Can you work these out from the model? Positions are in its coordinate system, mm. A direction names the side the tool comes from. Give positions to 0.01 mm unless a question says otherwise; leave off trailing zeros. Order: outer loops, then holes, each group sorted by start corner. A loop starts at its lowest first (then second) coordinate and runs counter-clockwise, first axis right, second up. Notation, with made-up numbers: (51, 73) - (104, 73) arc R33 ccw to (104, 110) - close; hole circle Ø10 at (29, 41.5). An arc over 180 degrees is marked (long way). Answer as CSV lines item,"result".
```python
from build123d import *

# Parameters (mm, degrees)
F0_W     = 62.4
F0_H     = 62.4
F0_W_2   = 60
F0_H_2   = 60
F1_DEPTH = 50


with BuildPart() as f1:
    # F0 (on Top) → F1 (new body)
    with BuildSketch(Plane.XY):
        Rectangle(F0_W, F0_H)
        Rectangle(F0_W_2, F0_H_2, mode=Mode.SUBTRACT)
    extrude(amount=F1_DEPTH)


solid = f1.part
```
1) I want a section at A-A on z = 23.5. Write out the boundary of the cut face in (x, y).
Answer block:
outline,"(-31.2, -31.2) - (31.2, -31.2) - (31.2, 31.2) - (-31.2, 31.2) - close; hole (-30, -30) - (30, -30) - (30, 30) - (-30, 30) - close"
2) If we mould it in two halves opening along Y, with no side actions, what happens to faces 3 (the flat face through (0, 30, 25)), 4 (the flat face through (-31.2, 0, 25)), 5 (the flat face through (-30, 0, 25)), 6 (the flat face through (0, -31.2, 25))? For each: +Y half, -Y half, draft (parallel to the pull), parting line (faces both ways), or undercut.
Answer block:
face 3,"undercut"
face 4,"draft"
face 5,"undercut"
face 6,"-Y half"
3) I'm going to push a flat-ended pin straight in: P1, Ø8, axis at x = -6.5, y = -22.5, coming from the +Z side. Where does the tip first touch, or does it pass through?
Answer block:
P1,"through"
4) I need wall thicknesses on line 1 along Y through (x, z) = (9, 10.5). Which ranges of the line are inside material? Lowest first, please. Write a range as [from, to].
Answer block:
line 1,"[-31.2, -30], [30, 31.2]"
5) I want a section at B-B on x = 5. Write out the boundary of the cut face in (y, z).
Answer block:
outline,"(-31.2, 0) - (-30, 0) - (-30, 50) - (-31.2, 50) - close; (30, 0) - (31.2, 0) - (31.2, 50) - (30, 50) - close"
6) Which directions (+Z, -Z, +X, -X, +Y, -Y) give clear straight access to the entire face, cutting with the end or side of a thin tool? Please do faces 1 (the flat face through (30, 0, 25)), 2 (the flat face through (-30.2, 14, 50)).
Answer block:
face 1,"+Z, -Z"
face 2,"+Z, +X, -X, +Y, -Y"
